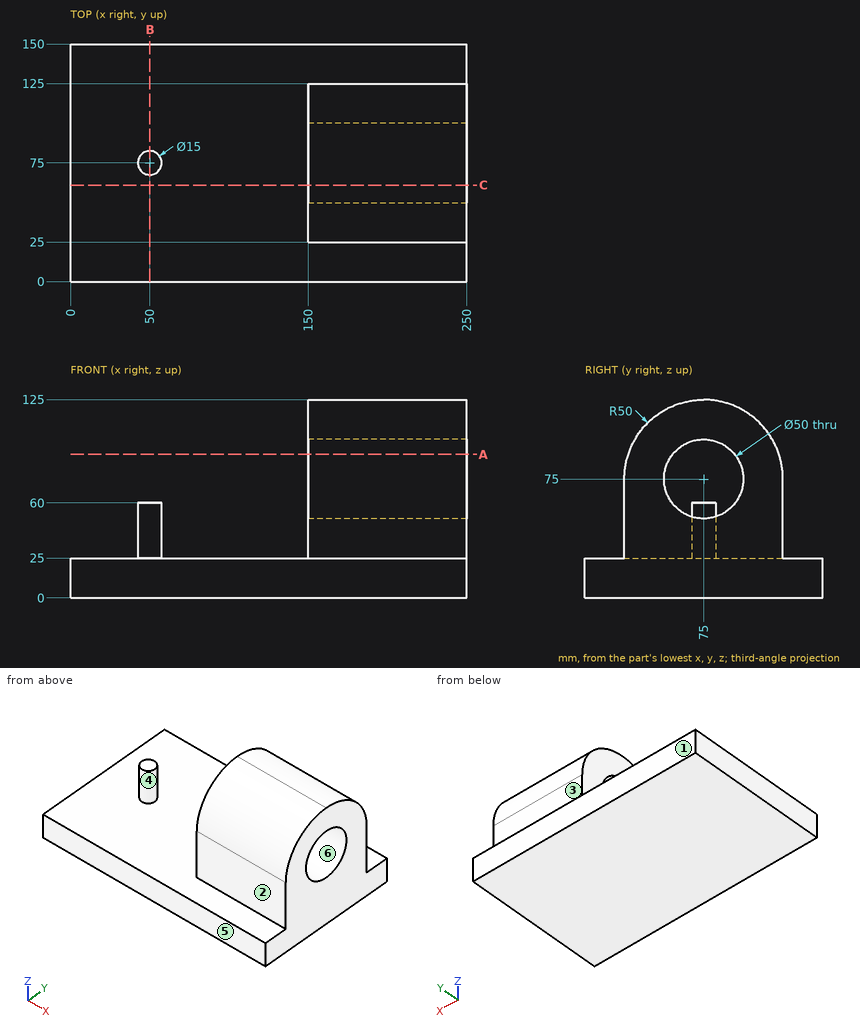
The figure shows three views and two pictorial views of one solid part (mm, origin at its lowest corner). Answer the questions. A direction names the side the tool comes from. Give positions to 0.01 mm unless a question says otherwise; leave off trailing zeros. Write each loop counter-clockwise with the first axis right and the second up, starting at its lowest first coordinate (ties: lowest second). Pieces come first, ordered by that corner, then holes. Notation, with made-up numbers: M 70,-24.5 L 80,-24.5 A19 ccw 80,-13.5 Z; hole C -4,28 d3. An arc over 180 degrees is marked long. One line per item, written item: value. Start each with the question number.
(1) Find section A-A (z = 90.5). Determine the outline of the cut face in (x, y).
(2) Find section B-B (x = 50). Determine the outline of the cut face in (y, z).
(3) Determine the mould class of the marked faces 4, 5 and 6 for opening direction Y: pulls with the +Y half, pulls with the -Y half, needs draft (parallel to the pull), parting line crosses it, or undercut.
(4) Find the intervals of material crossed by line 1 (X direction, y = 46, z = 50); line 2 (Z direction, x = 124.5, y = 121.5); line 3 (Y direction, x = 180, z = 61), in increasing order.
(5) Flat-ended cylindrical pins translate along their axes: pin 1 Ø1.5 at (y, z) = (127.5, 78) entering from -X; pin 2 Ø10 at (x, y) = (94, 70) entering from +Z; pin 3 Ø4 at (y, z) = (44, 52.5) entering from -X; pin 4 Ø15 at (x, z) = (214, 43.5) entering from -Y. Find the tip coordinate at first contact, or state that the pin passes through.
(6) Find section C-C (y = 61). Determine the outline of the cut face in (x, z).
(7) A tool of negligible diameter and unlimited length cuts with its end or side. For the marked faces 1, 2 and 3, from which of +Z, -Z, +X, -X, +Y, -Y can it reach the whole face along a straight path? Write none if from no direction.
Results below:
1. outline: M 150,27.46 L 250,27.46 L 250,55.38 L 150,55.38 Z; M 150,94.62 L 250,94.62 L 250,122.54 L 150,122.54 Z
2. outline: M 0,0 L 150,0 L 150,25 L 82.5,25 L 82.5,60 L 67.5,60 L 67.5,25 L 0,25 Z
3. face 4: parting line crosses it
3. face 5: pulls with the -Y half
3. face 6: undercut
4. line 1: x = 150 to 250
4. line 2: z = 0 to 25
4. line 3: y = 25 to 54.29, 95.71 to 125
5. pin 1: passes through
5. pin 2: stops at z = 25
5. pin 3: stops at x = 150
5. pin 4: stops at y = 25
6. outline: M 0,0 L 250,0 L 250,54.29 L 150,54.29 L 150,25 L 0,25 Z; M 150,95.71 L 250,95.71 L 250,123 L 150,123 Z
7. face 1: +Z, -Z, +X, -X, +Y
7. face 2: +Z, +X, -X, -Y
7. face 3: +Z, +X, -X, +Y
